Part model, mm, in its own coordinate system. Give positions to 0.01 mm unless a question says otherwise; leave off trailing zeros. Write each loop counter-clockwise with the first axis right and the second up, starting at its lowest first coordinate (ties: lowest second). Pieces come first, ordered by that corner, then holes. Notation, with made-up numbers: M 68,58 L 80,58 A21 cw 80,89 Z; hole C -20,25 d11. An arc over 180 degrees is marked long. Answer as CSV lines item,"result". Start each with the question number.
Item 1: Wall check: L1, parallel to Y at x = 0, z = 1.45; L2, parallel to X at y = -3.5, z = 0.8. Give the ranges that are in metal, low to high. Write a range as from..to.
Item 2: Band-saw the part on B-B, the plane y = -24. List the corners of the cut face in (x, z), then the cut area to 3 significant figures.
Item 3: Two-plate mould, pull along Y, no slides. Class faces 1 (the flat face through (48, 1, 1)), 2 (the flat face through (-11, -45, 3)): +Y half, -Y half, draft (parallel to the pull), parting line (faces both ways), or undercut.
Item 4: Band-saw the part on C-C, the plane z = 2.4. List the corners of the cut face in (x, y), then the cut area to 3 significant figures.
Item 5: Pin check, flat tips, straight feed: pin 1 (2 mm diameter, centred on x = -32, y = 29.5, fed in from -Z); pin 2 (1.5 mm diameter, centred on x = -31, z = 2.5, fed in from +Y); pin 3 (1 mm diameter, centred on y = 23.5, z = 0.5, fed in from +X). Stop position of each tip, or through.
Item 6: Band-saw the part on A-A, the plane x = 0. List the corners of the cut face in (y, z).
Solid Edge part; units mm, degrees
sketch "Sketch1" plane through (0, 0, 0) normal (0, 0, 1) x (1, 0, 0)
  circle A0 centre (0, 0) radius 46
  circle A1 centre (0, 0) radius 50.5
extrude "Protrusion1" add sketch "Sketch1" along normal blind 3
sketch "Sketch2" plane through (0, 0, 0) normal (1, 0, 0) x (0, 1, 0)
  line L0 (0, 0) -> (3, 3)
  line L1 (3, 3) -> (6, 3)
  line L2 (3, 0) -> (6, 3)
  line L3 (0, 0) -> (3, 0)
extrude "ExtrudedCutout_1" cut sketch "Sketch2" along normal blind 77.4946
properties part number "4" material "Cast Iron"
Output:
1,L1,"-50.5..-46, 46..50.5"
1,L2,"-50.38..-45.87, 45.87..50.38"
2,outline,"M -44.43,0 L -39.24,0 L -39.24,3 L -44.43,3 Z; M 39.24,0 L 44.43,0 L 44.43,3 L 39.24,3 Z"
2,area,"31.1 mm²"
3,face 1,"undercut"
3,face 2,"draft"
4,outline,"M 45.68,5.4 L 50.21,5.4 A50.5 ccw long 50.44,2.4 L 45.94,2.4 A46 cw long Z"
4,area,"1,350 mm²"
5,pin 1,"through"
5,pin 2,"y = 40.44"
5,pin 3,"x = 44.96"
6,outline,"M -50.5,0 L -46,0 L -46,3 L -50.5,3 Z; M 46,0 L 50.5,0 L 50.5,3 L 46,3 Z"
